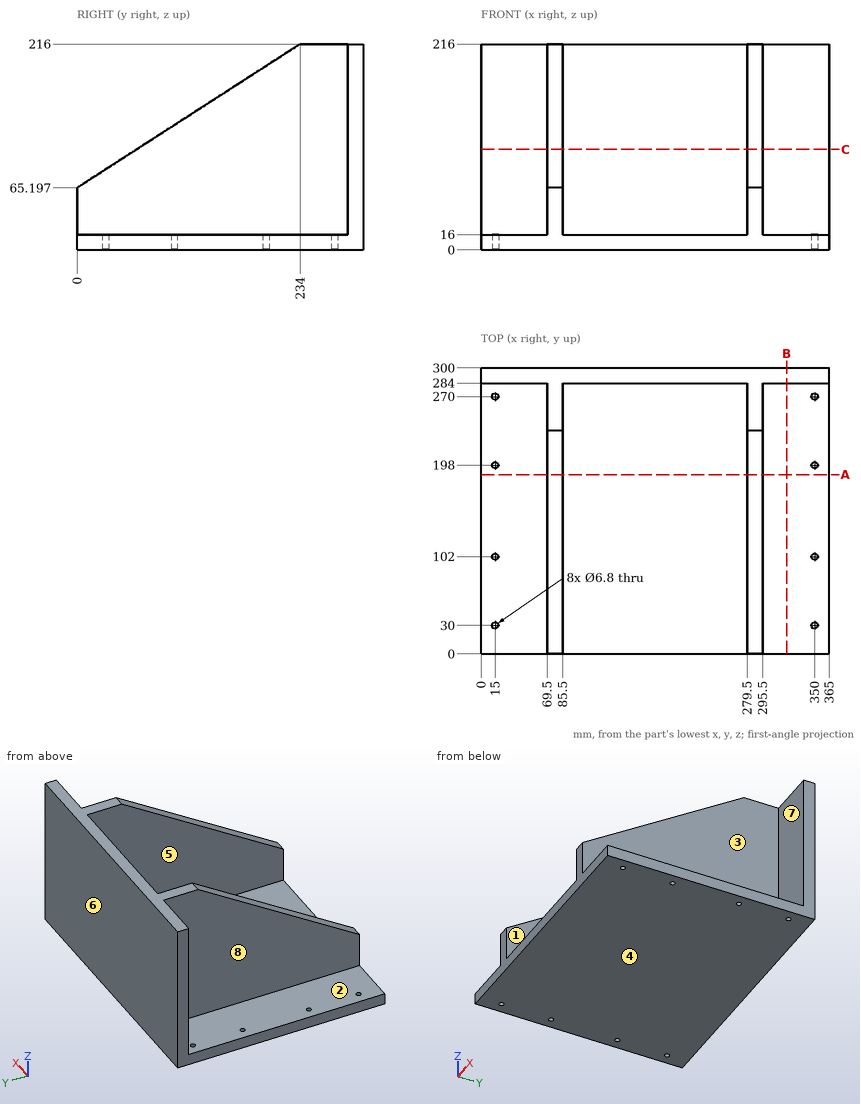
Drawing for the job (mm, zero at the part's lowest x, y, z). A direction names the side the tool comes from. Give positions to 0.01 mm unless a question says otherwise; leave off trailing zeros. Order: outer loops, then holes, each group sorted by start corner. A loop starts at its lowest first (then second) coordinate and runs counter-clockwise, first axis right, second up. Notation, with made-up numbers: M 33,76 L 61,76 A32 cw 61,109 Z; hole C -3,24 d6. An arc over 180 degrees is marked long. Use a Markdown table: item, result. Add a question column.
(1) Saw through at B-B, the plane x = 320.5. Give the cut face in (y, z), and give its area (3 significant figures).
(2) Mould opens along X. For the marked faces 1, 2 and 3 say: +X half, -X half, draft (parallel to the pull), parting line (faces both ways), or undercut.
(3) Drop flat-ended pins along their axis: P1, Ø21, axis at x = 344.5, y = 200, coming from the +Z side; P2, Ø12, axis at y = 229.5, z = 88.5, coming from the -X side. Give the stop position or say it passes through.
(4) Saw through at A-A, the plane y = 188. Give the cut face in (x, z) (1 decimal).
(5) Saw through at C-C, the plane z = 105.5. Give the cut face in (x, y), and give its area (3 significant figures).
(6) Probe line 1 along Y through (x, z) = (350, 9); line 2 along X through (y, z) = (198, 8); line 3 along X through (y, z) = (232, 53.5). List the from-to ranges inside material, lowest first. Write a range as [from, to].
(7) 3-axis set-ups, long thin cutter, end or side, ignore diameter. For the marked faces 4, 5, 6, 7 and 8: which of +Z, -Z, +X, -X, +Y, -Y reach the whole face in a straight line?
Answer key:
| question | item | result |
|---|---|---|
| 1 | outline | M 0,0 L 300,0 L 300,216 L 284,216 L 284,16 L 0,16 Z |
| 1 | area | 8,000 mm^2 |
| 2 | face 1 | undercut |
| 2 | face 2 | draft |
| 2 | face 3 | +X half |
| 3 | P1 | z = 16 |
| 3 | P2 | x = 69.5 |
| 4 | outline | M 0,0 L 365,0 L 365,16 L 295.5,16 L 295.5,186.4 L 279.5,186.4 L 279.5,16 L 85.5,16 L 85.5,186.4 L 69.5,186.4 L 69.5,16 L 0,16 Z |
| 5 | outline | M 0,284 L 69.5,284 L 69.5,62.54 L 85.5,62.54 L 85.5,284 L 279.5,284 L 279.5,62.54 L 295.5,62.54 L 295.5,284 L 365,284 L 365,300 L 0,300 Z |
| 5 | area | 12,900 mm^2 |
| 6 | line 1 | [0, 26.6], [33.4, 98.6], [105.4, 194.6], [201.4, 266.6], [273.4, 300] |
| 6 | line 2 | [0, 11.6], [18.4, 346.6], [353.4, 365] |
| 6 | line 3 | [69.5, 85.5], [279.5, 295.5] |
| 7 | face 4 | -Z, +X, -X, +Y, -Y |
| 7 | face 5 | +Z, -Y |
| 7 | face 6 | +Z, -Z, +X, -X, +Y |
| 7 | face 7 | +Z, +X, -Y |
| 7 | face 8 | +Z, -X, -Y |
